CAD build for the part. Positions are in the model's coordinates, mm. A direction names the side the tool comes from. Round coordinates to 2 decimals unless told otherwise and drop trailing zeros. Put each result on its own line as item: value.
```python
from build123d import *
from build123d.topology import SkipClean

# Parameters (mm, degrees)
SKETCH_1_R               = 26
EXTRUDE_1_DEPTH          = 10
EXTRUDE_2_DEPTH          = 12
EXTRUDE_3_DEPTH          = 4
EXTRUDE_4_DEPTH          = 8
EXTRUDE_START            = -15
EXTRUDE_5_DEPTH          = 33
SKETCH_6_R               = 3.5
CUT_EXTRUDE_1_DEPTH      = 271.867126097
SKETCH_7_R               = 16
CUT_EXTRUDE_2_DEPTH      = 275.960646248
CUT_EXTRUDE_3_DEPTH      = 275.341679271
CUT_EXTRUDE_3_DEPTH_BACK = 275.341679271
SKETCH_8_W               = 47.47924493
SKETCH_8_H               = 2
SKETCH_9_R               = 10
CUT_EXTRUDE_4_DEPTH      = 276.127892052
CHAMFER_1_SIZE           = 2
FILLET_1_R               = 2


# Read off the part's stored shape, not the designer's step: the hole wizard step
with BuildPart() as part:
    # Sketch 1 → Extrude 1 (new, symmetric)
    with BuildSketch(Plane(origin=(0, 0, 0), x_dir=(1, 0, 0), z_dir=(0, 1, 0))):
        with Locations(Location((0, 0, 0), (0, 0, 270))):
            Circle(SKETCH_1_R)
    extrude(amount=EXTRUDE_1_DEPTH, both=True)



with BuildPart() as body_2:
    # Sketch 2 → Extrude 2 (new, symmetric)
    with BuildSketch(Plane(origin=(0, 0, 0), x_dir=(1, 0, 0), z_dir=(0, 1, 0))):
        with BuildLine():
            Line((245, 16), (267, 16))
            Line((267, 16), (267, -16))
            Line((267, -16), (245, -16))
            ThreePointArc((245, -16), (229, 0), (245, 16))
        make_face()
    extrude(amount=EXTRUDE_2_DEPTH, both=True)


with BuildPart() as part_1:
    add(part.part)

    add(body_2.part)  # Extrude 3 merges body 2
    # Sketch 3 → Extrude 3 (add, symmetric)
    with BuildSketch(Plane(origin=(0, 0, 0), x_dir=(1, 0, 0), z_dir=(0, 1, 0))):
        with BuildLine():
            Line((245, -16), (257.248496817, -16))
            ThreePointArc((257.248496817, -16), (122.236247563, -61.840572391), (-14.536770014, -21.556491309))
            ThreePointArc((-14.536770014, -21.556491309), (20.358485161, -16.17195356), (17.708836414, 19.036730624))
            ThreePointArc((17.708836414, 19.036730624), (125.0222059, -25.075347424), (234.842372308, 12.362143814))
            ThreePointArc((234.842372308, 12.362143814), (229.936894394, -5.394705691), (245, -16))
        make_face()
    extrude(amount=EXTRUDE_3_DEPTH, both=True)

    # Sketch 4 → Extrude 4 (add, symmetric)
    with SkipClean():  # the faces are left unmerged after this step: merging them gives an invalid solid
        with BuildSketch(Plane(origin=(0, 0, 0), x_dir=(1, 0, 0), z_dir=(0, 1, 0))):
            with BuildLine():
                Line((257.248496817, -16), (245, -16))
                ThreePointArc((245, -16), (229.936894394, -5.394705691), (234.842372308, 12.362143814))
                ThreePointArc((234.842372308, 12.362143814), (125.0222059, -25.075347424), (17.708836414, 19.036730624))
                ThreePointArc((17.708836414, 19.036730624), (20.358485161, -16.17195356), (-14.536770014, -21.556491309))
                ThreePointArc((-14.536770014, -21.556491309), (122.236247563, -61.840572391), (257.248496817, -16))
            make_face()
            with BuildLine():
                ThreePointArc((224.078129878, -1.809792966), (229.571334836, -14.24627289), (241.531331279, -20.711550818))
                ThreePointArc((241.531331279, -20.711550818), (126.363618071, -56.716382465), (8.753490395, -29.738466771))
                ThreePointArc((8.753490395, -29.738466771), (25.337079445, -17.861478248), (30.950628442, 1.74888508))
                ThreePointArc((30.950628442, 1.74888508), (126.959850958, -30.124394673), (224.078129878, -1.809792966))
            make_face(mode=Mode.SUBTRACT)
        extrude(amount=EXTRUDE_4_DEPTH, both=True)
    add(part_1.part.scale(1), mode=Mode.REPLACE)  # the faces are merged on a copy

    # Sketch 5 → Extrude 5 (add)
    with BuildSketch(Plane.XY.offset(EXTRUDE_START)):
        with BuildLine():
            Line((0, -8), (-31, -8))
            ThreePointArc((-31, -8), (-39, 0), (-31, 8))
            Line((-31, 8), (0, 8))
            ThreePointArc((0, 8), (8, 0), (0, -8))
        make_face()
    extrude(amount=EXTRUDE_5_DEPTH)

    # Sketch 6 → Cut-Extrude 1 (cut, through all)
    with BuildSketch(Plane.XY.offset(18)):
        with Locations((-31, 0)):
            Circle(SKETCH_6_R)
    extrude(amount=-CUT_EXTRUDE_1_DEPTH, mode=Mode.SUBTRACT)

    # Sketch 7 → Cut-Extrude 2 (cut, through all)
    with BuildSketch(Plane(origin=(0, 10, 0), x_dir=(1, 0, 0), z_dir=(0, 1, 0))):
        with Locations(Location((0, 0, 0), (0, 0, 270))):
            Circle(SKETCH_7_R)
    extrude(amount=-CUT_EXTRUDE_2_DEPTH, mode=Mode.SUBTRACT)

    # Sketch 8 → Cut-Extrude 3 (cut, two sides: drawn at the far end of the back side and taken through both)
    with BuildSketch(Plane(origin=(0, 0, 0), x_dir=(1, 0, 0), z_dir=(0, 1, 0)).offset(-CUT_EXTRUDE_3_DEPTH_BACK)):
        with Locations((-23.739622465, 1)):
            Rectangle(SKETCH_8_W, SKETCH_8_H)
    extrude(amount=CUT_EXTRUDE_3_DEPTH + CUT_EXTRUDE_3_DEPTH_BACK, mode=Mode.SUBTRACT)

    # Sketch 9 → Cut-Extrude 4 (cut, through all)
    with BuildSketch(Plane(origin=(0, 12, 0), x_dir=(1, 0, 0), z_dir=(0, 1, 0))):
        with Locations(Location((245, 0, 0), (0, 0, 270))):
            Circle(SKETCH_9_R)
    extrude(amount=-CUT_EXTRUDE_4_DEPTH, mode=Mode.SUBTRACT)

    # Chamfer 1
    chamfer_1_edges = [part_1.edges().sort_by_distance(p)[0] for p in [
        (245, -12, -10),
        (245, 12, -10),
    ]]
    chamfer(chamfer_1_edges, length=CHAMFER_1_SIZE)

    # Fillet 1
    fillet_1_edges = [part_1.edges().sort_by_distance(p)[0] for p in [
        (25.337079445, -4, 17.861478248),
        (126.959850958, -4, 30.124394673),
        (229.571334836, -4, 14.24627289),
        (126.363618071, -4, 56.716382465),
        (126.363618071, 4, 56.716382465),
        (229.571334836, 4, 14.24627289),
        (126.959850958, 4, 30.124394673),
        (25.337079445, 4, 17.861478248),
    ]]
    fillet(fillet_1_edges, radius=FILLET_1_R)

    # 6.0mm _1 outline → 6.0mm _1 (revolve, cut)
    with BuildSketch(Plane.YX):
        Polygon((0, 254.53912622), (3, 254.53912622), (3, 264.113248654), (8, 267), (0, 267), align=None)
    revolve(axis=Axis((0, 0, 0), (1, 0, 0)), mode=Mode.SUBTRACT)


solid = part_1.part
```
Item 1: Mould opens along Z. For faces 1 (the cylindrical face through (126.681, 0.112, 25.118)), 2 (the flat face through (259, 0, 16)), 3 (the conical face through (264.294, 1.529, -2.939)) say: pulls with the +Z half, pulls with the -Z half, needs draft (parallel to the pull), parting line crosses it, or undercut.
Answers below:
face 1: pulls with the -Z half
face 2: pulls with the +Z half
face 3: undercut
Item 2: Probe line 1 along Y through (x, z) = (260, 0); line 2 along Y through (x, z) = (-31, -9); line 3 along X through (y, z) = (6.25, -14). List the from-to ranges inside material, lowest first. Write a range as [from, to].
Answers below:
line 1: [-12, -3], [3, 12]
line 2: [-8, -3.5], [3.5, 8]
line 3: [-35.99, -7.75], [7.75, 23.38], [237.25, 267]
Item 3: Tool access for faces 4 (the cylindrical face through (259, -3, 0)), 5 (the flat face through (-28, 8, 11)), 6 (the flat face through (12, 10, 11)): list every direction of +Z, -Z, +X, -X, +Y, -Y with a clear straight run to the whole face (end or side of a thin tool).
Answers below:
face 4: +X
face 5: +Z, -X, +Y
face 6: +Z, -Z, -X, +Y
Item 4: Pin check, flat tips, straight feed: P1, Ø10, axis at x = 60, y = 3, coming from the -Z side; P2, Ø3, axis at x = 17, y = 7, coming from the -Z side; P3, Ø8, axis at x = -31, y = 0, coming from the +Z side; P4, Ø12, axis at y = -2, z = 6.5, coming from the +X side. Stop position of each tip, or through.
Answers below:
P1: z = 7.08
P2: z = -20.87
P3: z = 18
P4: x = 267
Item 5: Band-saw the part on A-A on y = 0. State how many separate pieces and enclosed holes the cut face has, and give its area (3 significant figures).
Answers below:
separate pieces: 3
enclosed holes: 0
area: 11,200 mm²
